```python
from build123d import *

# Parameters (mm, degrees)
SKETCH_1_W          = 81
SKETCH_1_H          = 60
SKETCH_1_W_2        = 10
SKETCH_1_H_2        = 3
SKETCH_1_W_3        = 3
SKETCH_1_H_3        = 10
EXTRUDE_1_DEPTH     = 3
CUT_EXTRUDE_1_DEPTH = 10


with BuildPart() as part:
    # 草图1 → 凸台-拉伸1 (new body)
    with BuildSketch(Plane.XY):
        Rectangle(SKETCH_1_W, SKETCH_1_H)
        with Locations((-30.5, 26.5)):
            Rectangle(SKETCH_1_W_2, SKETCH_1_H_2, mode=Mode.SUBTRACT)
        with Locations((-37, 15)):
            Rectangle(SKETCH_1_W_3, SKETCH_1_H_3, mode=Mode.SUBTRACT)
        with Locations((-37, 0)):
            Rectangle(SKETCH_1_W_3, SKETCH_1_H_3, mode=Mode.SUBTRACT)
        with Locations((-37, -15)):
            Rectangle(SKETCH_1_W_3, SKETCH_1_H_3, mode=Mode.SUBTRACT)
        with Locations((37, -15)):
            Rectangle(SKETCH_1_W_3, SKETCH_1_H_3, mode=Mode.SUBTRACT)
        with Locations((37, 0)):
            Rectangle(SKETCH_1_W_3, SKETCH_1_H_3, mode=Mode.SUBTRACT)
        with Locations((37, 15)):
            Rectangle(SKETCH_1_W_3, SKETCH_1_H_3, mode=Mode.SUBTRACT)
        with Locations((-15.5, 26.5)):
            Rectangle(SKETCH_1_W_2, SKETCH_1_H_2, mode=Mode.SUBTRACT)
        with Locations((-0.5, 26.5)):
            Rectangle(SKETCH_1_W_2, SKETCH_1_H_2, mode=Mode.SUBTRACT)
        with Locations((14.5, 26.5)):
            Rectangle(SKETCH_1_W_2, SKETCH_1_H_2, mode=Mode.SUBTRACT)
        with Locations((29.5, 26.5)):
            Rectangle(SKETCH_1_W_2, SKETCH_1_H_2, mode=Mode.SUBTRACT)
        with Locations((29.5, -26.5)):
            Rectangle(SKETCH_1_W_2, SKETCH_1_H_2, mode=Mode.SUBTRACT)
        with Locations((14.5, -26.5)):
            Rectangle(SKETCH_1_W_2, SKETCH_1_H_2, mode=Mode.SUBTRACT)
        with Locations((-0.5, -26.5)):
            Rectangle(SKETCH_1_W_2, SKETCH_1_H_2, mode=Mode.SUBTRACT)
        with Locations((-15.5, -26.5)):
            Rectangle(SKETCH_1_W_2, SKETCH_1_H_2, mode=Mode.SUBTRACT)
        with Locations((-30.5, -26.5)):
            Rectangle(SKETCH_1_W_2, SKETCH_1_H_2, mode=Mode.SUBTRACT)
    extrude(amount=EXTRUDE_1_DEPTH)

    # 草图2 → 切除-拉伸1 (cut)
    with BuildSketch(Plane.XY.offset(3)):
        Polygon((-27, 23), (27, 23), (0, 3), align=None)
        Polygon((-27, -23), (0, -3), (27, -23), align=None)
        Polygon((33, 21), (33, -21), (4.65, 0), align=None)
        Polygon((-33, 21), (-4.65, 0), (-33, -21), align=None)
    extrude(amount=-CUT_EXTRUDE_1_DEPTH, mode=Mode.SUBTRACT)


solid = part.part
```
Can you work these out from the model? Positions are in its coordinate system, mm. Coordinates: 2 decimals unless noted, no trailing zeros. Loops run counter-clockwise (first coordinate to the right, second up) from the corner with the lowest first, then second, coordinate; pieces in that order, holes last. Notation, with made-up numbers: (-18, 81) -> (-14, 81) arc R15 cw to (-14, 86) -> close; hole circle Ø7 at (9, 14). An arc over 180 degrees is marked (long way). Put each result on its own line as item: value. Start each with the question number.
Q1. I want a section at A-A (y = -22). Write out the boundary of the cut face in (x, z), plus the area to 3 significant figures.
Q2. Thinking about a two-plate mould opening in X: for faces 1 (the face through (-1, 0, 0)), 2 (the face through (37, 5, 1)), which applies, pulls with the +X half, pulls with the -X half, needs draft (parallel to the pull), parting line crosses it, or undercut?
Q3. I want a section at B-B (x = -34). Write out the boundary of the cut face in (y, z), plus the area to 3 significant figures.
Q4. If I drill on line 1 (Y direction, x = -35, z = 1.1); line 2 (Y direction, x = 29, z = 2.55); line 3 (X direction, y = 12, z = 0.35), over which ranges is the centre line in solid material (lowest first)? Write a range as [from, to].
Q5. I want a section at C-C (y = 12). Write out the boundary of the cut face in (x, z), plus the area to 3 significant figures.
Q6. I want a section at D-D (x = 13.5). Write out the boundary of the cut face in (y, z), plus the area to 3 significant figures.
Taken from the geometry:
1. outline: (-40.5, 0) -> (-25.65, 0) -> (-25.65, 3) -> (-40.5, 3) -> close; (25.65, 0) -> (40.5, 0) -> (40.5, 3) -> (25.65, 3) -> close
1. area: 89.1 mm2
2. face 1: needs draft
2. face 2: undercut
3. outline: (-30, 0) -> (-28, 0) -> (-28, 3) -> (-30, 3) -> close; (-25, 0) -> (25, 0) -> (25, 3) -> (-25, 3) -> close; (28, 0) -> (30, 0) -> (30, 3) -> (28, 3) -> close
3. area: 162 mm2
4. line 1: y = [-30, -28], [-25, 25], [28, 30]
4. line 2: y = [-30, -28], [-25, -18.04], [18.04, 25], [28, 30]
4. line 3: x = [-40.5, -38.5], [-35.5, -33], [-20.85, -12.15], [12.15, 20.85], [33, 35.5], [38.5, 40.5]
5. outline: (-40.5, 0) -> (-38.5, 0) -> (-38.5, 3) -> (-40.5, 3) -> close; (-35.5, 0) -> (-33, 0) -> (-33, 3) -> (-35.5, 3) -> close; (-20.85, 0) -> (-12.15, 0) -> (-12.15, 3) -> (-20.85, 3) -> close; (12.15, 0) -> (20.85, 0) -> (20.85, 3) -> (12.15, 3) -> close; (33, 0) -> (35.5, 0) -> (35.5, 3) -> (33, 3) -> close; (38.5, 0) -> (40.5, 0) -> (40.5, 3) -> (38.5, 3) -> close
5. area: 79.2 mm2
6. outline: (-30, 0) -> (-28, 0) -> (-28, 3) -> (-30, 3) -> close; (-25, 0) -> (-23, 0) -> (-23, 3) -> (-25, 3) -> close; (-13, 0) -> (-6.56, 0) -> (-6.56, 3) -> (-13, 3) -> close; (6.56, 0) -> (13, 0) -> (13, 3) -> (6.56, 3) -> close; (23, 0) -> (25, 0) -> (25, 3) -> (23, 3) -> close; (28, 0) -> (30, 0) -> (30, 3) -> (28, 3) -> close
6. area: 62.7 mm2
